Check sheet for the modelled part. Datum: model origin and axes. Units: mm. A direction names the side the tool comes from. Round coordinates to 2 decimals unless told otherwise and drop trailing zeros. Loops run counter-clockwise (first coordinate to the right, second up) from the corner with the lowest first, then second, coordinate; pieces in that order, holes last. Notation, with made-up numbers: (-28, -8) - (-23, -8) arc R18 ccw to (-23, 1) - close; hole circle Ø1 at (-23.5, 82). An arc over 180 degrees is marked (long way). Answer in a Markdown table with one row per item. Add a question column.
(1) Cross-section at B-B on z = 93. Enter the section's corners in (x, y), then the cut area to 3 significant figures.
(2) Mould release check, pull along Z, two halves, no side actions. Record for faces 6 (the flat face through (2.7, 21.5, 109)), 7 (the flat face through (0, 15, 3)), 8 (the flat face through (23, 13, 6)): +Z half, -Z half, draft (parallel to the pull), parting line (faces both ways), or undercut.
(3) Gauge pin test, flat ends, axial feed: pin 1 (8 mm diameter, centred on x = 23, z = 9.5, fed in from +Y); pin 2 (3 mm diameter, centred on x = 12.5, z = 51, fed in from +Y); pin 3 (0.8 mm diameter, centred on x = 31, y = 22, fed in from +Z). Record the tip position at first contact, or that the pin passes through.
(4) Thickness scan on line 1 along X through (y, z) = (17.5, 85.5); line 2 along Z through (x, y) = (13, 20.75); line 3 along X through (y, z) = (12.5, 74). Record the ranges inside material, lowest first.
(5) Cross-section at D-D on z = 105.5. Enter the section's corners in (x, y).
(6) Cross-section at A-A on x = 30. Enter the section's corners in (y, z).
(7) Access from +Z, -Z, +X, -X, +Y, -Y to the whole of each face (thin tool, end or side, straight path). Record for faces 1 (the cylindrical face through (1.203, 20.359, 2.958)), 2 (the cylindrical face through (23.1, 4.2, 12.5)), 3 (the flat face through (19, 21.5, 112)), 4 (the cylindrical face through (3.379, 11.744, 56.779)), 5 (the flat face through (19, 21.5, 3)).
(8) Cross-section at C-C on y = 1.75. Enter the section's corners in (x, z), then the cut area to 3 significant figures.
from build123d import *
from OCP.BRepFilletAPI import BRepFilletAPI_MakeChamfer

# Parameters (mm, degrees)
SCHIZZO1_W               = 37
SCHIZZO1_H               = 21.5
ESTRUSIONE1_DEPTH        = 115
SCHIZZO6_W               = 103
SCHIZZO6_H               = 23.639461627
TAGLIO_ESTRUSIONE4_DEPTH = 84
SCHIZZO7_R               = 5.5
ESTRUSIONE4_DEPTH        = 103
SMUSSO1_SIZE             = 3
SMUSSO1_SIZE2            = 0.803847577
RACCORDO1_R              = 4
SCHIZZO8_R               = 45
TAGLIO_ESTRUSIONE5_DEPTH = 123.883074506
SCHIZZO9_R               = 3
TAGLIO_ESTRUSIONE6_DEPTH = 8.5


with BuildPart() as part:
    # Schizzo1 → Estrusione1 (new body)
    with BuildSketch(Plane.XY):
        with Locations((18.5, 10.75)):
            Rectangle(SCHIZZO1_W, SCHIZZO1_H)
    extrude(amount=ESTRUSIONE1_DEPTH)

    # Schizzo6 → Taglio-Estrusione4 (cut)
    with BuildSketch(Plane(origin=(37, 0, 0), x_dir=(0, 0, -1), z_dir=(1, 0, 0))):
        with Locations((-57.5, 20.319730814)):
            Rectangle(SCHIZZO6_W, SCHIZZO6_H)
    extrude(amount=-TAGLIO_ESTRUSIONE4_DEPTH, mode=Mode.SUBTRACT)

    # Schizzo7 → Estrusione4 (add)
    with BuildSketch(Plane.XY.offset(6)):
        with Locations(Location((5, 17, 0), (0, 0, 155.380022671))):
            Circle(SCHIZZO7_R)
        with Locations(Location((17.5, 17, 0), (0, 0, 125.096801228))):
            Circle(SCHIZZO7_R)
        with Locations(Location((30, 17, 0), (0, 0, 125.096801228))):
            Circle(SCHIZZO7_R)
    extrude(amount=ESTRUSIONE4_DEPTH)

    # Smusso1: one chamfer whose edges measure the first distance from different faces: ONE call of the kernel's chamfer builder (chamfer() names one face for all edges)
    smusso1_edges_1 = [part.edges().sort_by_distance(p)[0] for p in [
        (37, 21.5, 3),
    ]]
    smusso1_side_1 = [part.faces().sort_by_distance(p)[0] for p in [
        (18.5, 21.5, 3),
    ]]
    smusso1_edges_2 = [part.edges().sort_by_distance(p)[0] for p in [
        (37, 21.5, 112),
    ]]
    smusso1_side_2 = [part.faces().sort_by_distance(p)[0] for p in [
        (18.5, 21.5, 112),
    ]]
    smusso1 = BRepFilletAPI_MakeChamfer(part.part.solid().wrapped)
    for e in smusso1_edges_1:
        smusso1.Add(SMUSSO1_SIZE, SMUSSO1_SIZE2, e.wrapped, smusso1_side_1[0].wrapped)  # the first distance lies on this face
    for e in smusso1_edges_2:
        smusso1.Add(SMUSSO1_SIZE, SMUSSO1_SIZE2, e.wrapped, smusso1_side_2[0].wrapped)  # the first distance lies on this face
    add(Compound.cast(smusso1.Shape()), mode=Mode.REPLACE)

    # Raccordo1
    # the kernel refuses this fillet: 4 mm, written as the material it takes off along each edge
    with BuildSketch(Plane(origin=(0, 21.5, -10), x_dir=(1, 0, 0), z_dir=(0, 0, 1))) as raccordo1_piece_1:
        with BuildLine():
            CenterArc((RACCORDO1_R, -RACCORDO1_R), RACCORDO1_R, 90, 90)
            Line((0, -RACCORDO1_R), (0, 0))
            Line((0, 0), (RACCORDO1_R, 0))
        make_face()
    extrude(amount=16, mode=Mode.SUBTRACT)
    with BuildSketch(Plane(origin=(0, 21.5, 109), x_dir=(0, -1, 0), z_dir=(0, 0, 1))) as raccordo1_piece_2:
        with BuildLine():
            CenterArc((RACCORDO1_R, RACCORDO1_R), RACCORDO1_R, 180, 90)
            Line((0, RACCORDO1_R), (0, 0))
            Line((0, 0), (RACCORDO1_R, 0))
        make_face()
    extrude(amount=16, mode=Mode.SUBTRACT)

    # Schizzo8 → Taglio-Estrusione5 (cut, through all)
    with BuildSketch(Plane.XY.offset(115)):
        with Locations((-24.5, -24.5)):
            Circle(SCHIZZO8_R)
    extrude(amount=-TAGLIO_ESTRUSIONE5_DEPTH, mode=Mode.SUBTRACT)

    # Schizzo9 → Taglio-Estrusione6 (cut)
    with BuildSketch(Plane.XZ):
        with Locations(Location((23, 105.5, 0), (0, 0, 270))):
            Circle(SCHIZZO9_R)
        with Locations(Location((23, 9.5, 0), (0, 0, 270))):
            Circle(SCHIZZO9_R)
    extrude(amount=-TAGLIO_ESTRUSIONE6_DEPTH, mode=Mode.SUBTRACT)


solid = part.part
Answers:
| question | item | result |
|---|---|---|
| 1 | outline | circle Ø11 at (5, 17); (6.09, 8.5) arc R45 cw to (13.25, 0) - (37, 0) - (37, 8.5) - close; circle Ø11 at (17.5, 17); circle Ø11 at (30, 17) |
| 1 | area | 515 mm^2 |
| 2 | face 6 | +Z half |
| 2 | face 7 | draft |
| 2 | face 8 | undercut |
| 3 | pin 1 | stops at y = 22.29 |
| 3 | pin 2 | stops at y = 21.24 |
| 3 | pin 3 | stops at z = 109 |
| 4 | line 1 | x = -0.48 to 10.48, 12.02 to 22.98, 24.52 to 35.48 |
| 4 | line 2 | z = 0 to 6, 109 to 115 |
| 4 | line 3 | x = 1.84 to 8.16, 14.34 to 20.66, 26.84 to 33.16 |
| 5 | outline | circle Ø11 at (5, 17); (6.09, 8.5) arc R45 cw to (13.25, 0) - (20, 0) - (20, 8.5) - close; circle Ø11 at (17.5, 17); circle Ø11 at (30, 17); (26, 0) - (37, 0) - (37, 8.5) - (26, 8.5) - close |
| 6 | outline | (0, 0) - (21.5, 0) - (21.5, 6) - (22.5, 6) - (22.5, 109) - (21.5, 109) - (21.5, 115) - (0, 115) - close; hole (8.5, 6) - (11.5, 6) - (11.5, 109) - (8.5, 109) - close |
| 7 | face 1 | -Z, -X, +Y |
| 7 | face 2 | -Y |
| 7 | face 3 | +Z, +X, -X, +Y |
| 7 | face 4 | none |
| 7 | face 5 | -Z, +X, -X, +Y |
| 8 | outline | (12.05, 0) - (37, 0) - (37, 115) - (12.05, 115) - close; hole circle Ø6 at (23, 9.5); hole circle Ø6 at (23, 105.5) |
| 8 | area | 2,810 mm^2 |
